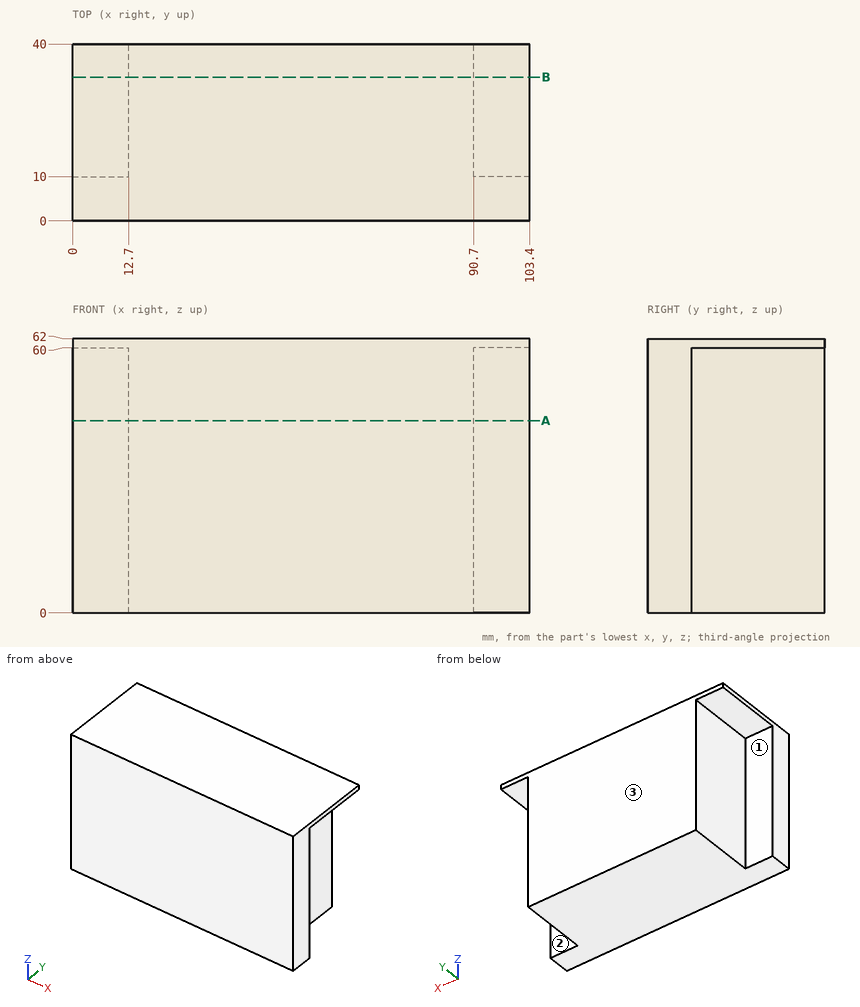
Source: three-view drawing plus pictorial views. Frame: mm from the lowest corner of the part. A direction names the side the tool comes from. Round coordinates to 2 decimals unless told otherwise and drop trailing zeros. Loops run counter-clockwise (first coordinate to the right, second up) from the corner with the lowest first, then second, coordinate; pieces in that order, holes last.
1. Section query B-B on y = 32.5. Output: boundary loops of the cut face in (x, z), and give its area (3 significant figures).
2. Contact query for flat-ended pins moving along their axis: pin 1 (24 mm diameter, centred on y = 31.5, z = 44.5, fed in from -X); pin 2 (4 mm diameter, centred on x = 99.5, z = 30, fed in from +Y); pin 3 (4 mm diameter, centred on x = 8.5, y = 26.5, fed in from -Z). Output: stop coordinate, or through.
3. Section query A-A on z = 43.5. Output: boundary loops of the cut face in (x, y), and give its area (3 significant figures).
4. Access query for the marked faces 1, 2 and 3. Directions: +Z, -Z, +X, -X, +Y, -Y. A direction counts if a zero-diameter tool reaches every point of the face in a straight line with its end or side. Return the directions, or none.
5. Ray query, L1, parallel to Y at x = 98, z = 17.5; L2, parallel to X at y = 22, z = 32; L3, parallel to Z at x = 98.5, y = 21.5. Return the intervals inside material, ascending.
Answers below:
1. outline: (0, 60) - (12.7, 60) - (12.7, 0) - (90.7, 0) - (90.7, 60) - (103.4, 60) - (103.4, 62) - (0, 62) - close
1. area: 4,890 mm2
2. pin 1: stops at x = 12.7
2. pin 2: stops at y = 10
2. pin 3: stops at z = 60
3. outline: (0, 0) - (103.4, 0) - (103.4, 10) - (90.7, 10) - (90.7, 40) - (12.7, 40) - (12.7, 10) - (0, 10) - close
3. area: 3,370 mm2
4. face 1: -Z, -X, +Y
4. face 2: -Z, +X, +Y
4. face 3: +Z, -Z, +X, -X, +Y
5. L1: y = 0 to 10
5. L2: x = 12.7 to 90.7
5. L3: z = 60 to 62
